Geometry check sheet. Reference: the model listing, model coordinates, mm. Face numbers are marked on the shaded views. A direction names the side the tool comes from. Coordinates: 2 decimals unless noted, no trailing zeros. Loops run counter-clockwise (first coordinate to the right, second up) from the corner with the lowest first, then second, coordinate; pieces in that order, holes last. Notation, with made-up numbers: M 70,35.25 L 87,35.25 A15 ccw 87,55.25 Z; hole C 9,12 d10. An arc over 180 degrees is marked long. Use CSV: the item, a comma, the result in double quotes.
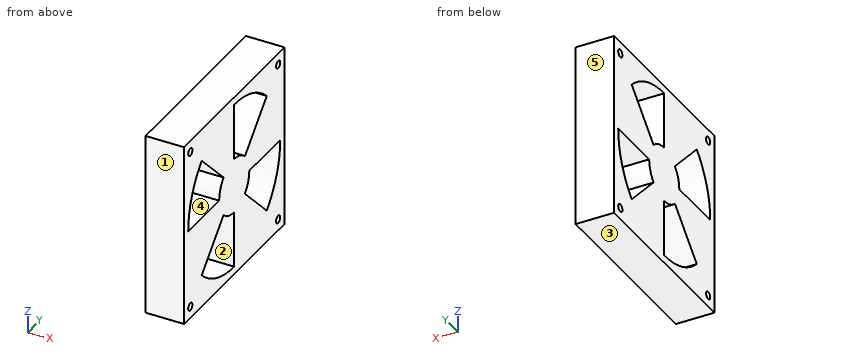
```python
from build123d import *

# Parameters (mm, degrees)
SKETCH_1_W      = 120
SKETCH_1_H      = 120
SKETCH_1_R      = 2.5
SKETCH_1_R_2    = 55
SKETCH_1_R_3    = 18
EXTRUDE_1_DEPTH = 25


with BuildPart() as part:
    # 草图1 → 凸台-拉伸1 (new body)
    # profile 1 of 6: a face of its own
    with BuildSketch(Plane(origin=(0, 0, 0), x_dir=(0, 0, -1), z_dir=(1, 0, 0))):
        with Locations((60, -60)):
            Rectangle(SKETCH_1_W, SKETCH_1_H)
        with Locations((7.5, -112.5)):
            Circle(SKETCH_1_R, mode=Mode.SUBTRACT)
        with Locations((112.5, -112.5)):
            Circle(SKETCH_1_R, mode=Mode.SUBTRACT)
        with Locations((112.5, -7.5)):
            Circle(SKETCH_1_R, mode=Mode.SUBTRACT)
        with Locations((7.5, -7.5)):
            Circle(SKETCH_1_R, mode=Mode.SUBTRACT)
        with Locations((60, -60)):
            Circle(SKETCH_1_R_2, mode=Mode.SUBTRACT)
    # profile 2 of 6: a face of its own
    with BuildSketch(Plane(origin=(0, 0, 0), x_dir=(0, 0, -1), z_dir=(1, 0, 0))):
        with Locations((60, -60)):
            Circle(SKETCH_1_R_3)
    # profile 3 of 6: a face of its own
    with BuildSketch(Plane(origin=(0, 0, 0), x_dir=(0, 0, -1), z_dir=(1, 0, 0))):
        with BuildLine():
            ThreePointArc((47.272077939, -47.272077939), (53.111698217, -43.370168415), (60, -42))
            Line((60, -42), (60, -5))
            ThreePointArc((60, -5), (38.95241122, -9.186625712), (21.109127035, -21.109127035))
            Line((21.109127035, -21.109127035), (47.272077939, -47.272077939))
        make_face()
    # profile 4 of 6: a face of its own
    with BuildSketch(Plane(origin=(0, 0, 0), x_dir=(0, 0, -1), z_dir=(1, 0, 0))):
        with BuildLine():
            Line((98.890872965, -21.109127035), (72.727922061, -47.272077939))
            ThreePointArc((72.727922061, -47.272077939), (76.629831585, -53.111698217), (78, -60))
            Line((78, -60), (115, -60))
            ThreePointArc((115, -60), (110.813374288, -38.95241122), (98.890872965, -21.109127035))
        make_face()
    # profile 5 of 6: a face of its own
    with BuildSketch(Plane(origin=(0, 0, 0), x_dir=(0, 0, -1), z_dir=(1, 0, 0))):
        with BuildLine():
            Line((98.890872965, -98.890872965), (72.727922061, -72.727922061))
            ThreePointArc((72.727922061, -72.727922061), (66.888301783, -76.629831585), (60, -78))
            Line((60, -78), (60, -115))
            ThreePointArc((60, -115), (81.04758878, -110.813374288), (98.890872965, -98.890872965))
        make_face()
    # profile 6 of 6: a face of its own
    with BuildSketch(Plane(origin=(0, 0, 0), x_dir=(0, 0, -1), z_dir=(1, 0, 0))):
        with BuildLine():
            ThreePointArc((47.272077939, -72.727922061), (43.370168415, -66.888301783), (42, -60))
            Line((42, -60), (5, -60))
            ThreePointArc((5, -60), (9.186625712, -81.04758878), (21.109127035, -98.890872965))
            Line((21.109127035, -98.890872965), (47.272077939, -72.727922061))
        make_face()
    extrude(amount=EXTRUDE_1_DEPTH)


solid = part.part
```
1. Set-up check for the marked faces 1 and 2: record each of +Z, -Z, +X, -X, +Y, -Y from which the full face is reachable in a straight line by a thin tool's end or side.
The answers:
face 1,"+Z, -Z, +X, -X, -Y"
face 2,"+X, -X"
2. Section check B-B, the plane y = -24. Record the cut outline in (x, z).
The answers:
outline,"M 0,-120 L 25,-120 L 25,-96 L 0,-96 Z; M 0,-60 L 25,-60 L 25,-24 L 0,-24 Z; M 0,-18.42 L 25,-18.42 L 25,0 L 0,0 Z"
3. Gauge pin test, flat end, axial feed: P1, Ø10, axis at x = 12, y = -92.5, coming from the +Z side. Record the tip position at first contact, or that the pin passes through.
The answers:
P1,"z = 0"
4. Section check C-C, the plane x = 23.5. Count the separate pieces of the cut face and the enclosed holes in it, plus the area to 3 significant figures.
The answers:
separate pieces,"1"
enclosed holes,"8"
area,"10,100 mm^2"
5. Thickness scan on line 1 (Y direction, x = 21.5, z = -92); line 2 (Y direction, x = 11.5, z = -46.5); line 3 (Z direction, x = 7.5, y = -36.5). Record the ranges inside material, lowest first. Write a range as [from, to].
The answers:
line 1,"[-120, -92], [-60, -28], [-15.27, 0]"
line 2,"[-120, -113.32], [-73.5, -48.09], [-46.5, 0]"
line 3,"[-120, -83.5], [-60, -36.5], [-10.27, 0]"
6. Release check for a two-part mould opening along Z. For the marked faces 3, 4 and 5 record: +Z half, -Z half, draft (parallel to the pull), parting line (faces both ways), or undercut.
The answers:
face 3,"-Z half"
face 4,"undercut"
face 5,"draft"
7. Section check D-D, the plane z = -112.5. Record the cut outline in (x, y).
The answers:
outline,"M 0,-120 L 25,-120 L 25,-115 L 0,-115 Z; M 0,-110 L 25,-110 L 25,-76.39 L 0,-76.39 Z; M 0,-60 L 25,-60 L 25,-10 L 0,-10 Z; M 0,-5 L 25,-5 L 25,0 L 0,0 Z"
8. Section check A-A, the plane z = -16. Record the cut outline in (x, y), plus the area to 4 significant figures.
The answers:
outline,"M 0,-120 L 25,-120 L 25,-60 L 0,-60 Z; M 0,-27 L 25,-27 L 25,0 L 0,0 Z"
area,"2,175 mm^2"
